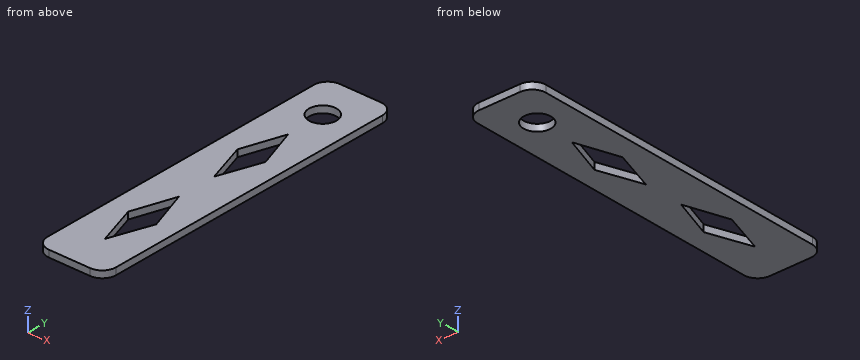
```python
from build123d import *

# Parameters (mm, degrees)
F0_R     = 12.7
F1_DEPTH = 6.35


with BuildPart() as f1:
    # F0 (on Top) → F1 (new body)
    with BuildSketch(Plane.XY):
        with BuildLine():
            ThreePointArc((0, 12.7), (3.719744, 3.719744), (12.7, 0))
            Line((12.7, 0), (50.8, 0))
            ThreePointArc((50.8, 0), (59.780256, 3.719744), (63.5, 12.7))
            Line((63.5, 12.7), (63.5, 292.1))
            ThreePointArc((63.5, 292.1), (59.780256, 301.080256), (50.8, 304.8))
            Line((50.8, 304.8), (12.7, 304.8))
            ThreePointArc((12.7, 304.8), (3.719744, 301.080256), (0, 292.1))
            Line((0, 292.1), (0, 12.7))
        make_face()
        Polygon((19.05, 75.692), (31.75, 114.540583), (45.188366, 75.692), (31.75, 36.843417), align=None, mode=Mode.SUBTRACT)
        Polygon((19.05, 190.246), (31.75, 229.094583), (45.188366, 190.246), (31.75, 151.397417), align=None, mode=Mode.SUBTRACT)
        with Locations((31.75, 265.397549)):
            Circle(F0_R, mode=Mode.SUBTRACT)
    extrude(amount=F1_DEPTH)


solid = f1.part
```
The listing builds one solid part. Answer for the finished solid, in the listing's coordinates (mm). Give positions to 0.01 mm unless a question says otherwise; leave off trailing zeros. Order: outer loops, then holes, each group sorted by start corner. A loop starts at its lowest first (then second) coordinate and runs counter-clockwise, first axis right, second up. Notation, with made-up numbers: (1, -38) -> (7, -38) arc R31 cw to (7, -13) -> close; hole circle Ø1 at (-32.5, -14). An arc over 180 degrees is marked (long way). Write each question's results on one line, items separated by ' | '.
Q1. The part is cut by section B-B, the plane y = 108.5. Give the vertices of the cut face in (x, z), and give its area (3 significant figures).
Checked values:
outline: (0, 0) -> (29.78, 0) -> (29.78, 6.35) -> (0, 6.35) -> close; (33.84, 0) -> (63.5, 0) -> (63.5, 6.35) -> (33.84, 6.35) -> close | area: 377 mm^2
Q2. Each of these flat-tipped pins is pushed along its axis until it touches: P1, Ø3, axis at x = 29.5, y = 53, coming from the +Z side; P2, Ø6, axis at x = 33.5, y = 100.5, coming from the -Z side; P3, Ø2, axis at x = 10, z = 1.5, coming from the -Y side. Where does it stop, or does it pass through?
Checked values:
P1: passes through | P2: stops at z = 0 | P3: stops at y = 0.11
Q3. The part is cut by section A-A, the plane x = 37. Give the vertices of the cut face in (y, z).
Checked values:
outline: (0, 0) -> (52.02, 0) -> (52.02, 6.35) -> (0, 6.35) -> close; (99.36, 0) -> (166.57, 0) -> (166.57, 6.35) -> (99.36, 6.35) -> close; (213.92, 0) -> (253.83, 0) -> (253.83, 6.35) -> (213.92, 6.35) -> close; (276.96, 0) -> (304.8, 0) -> (304.8, 6.35) -> (276.96, 6.35) -> close
Q4. The part is cut by section D-D, the plane y = 260. Give the vertices of the cut face in (x, z).
Checked values:
outline: (0, 0) -> (20.25, 0) -> (20.25, 6.35) -> (0, 6.35) -> close; (43.25, 0) -> (63.5, 0) -> (63.5, 6.35) -> (43.25, 6.35) -> close
Q5. Straight lines are drawn through the part: probe 1 along X at (y, z) = (196.5, 4) (1 decimal); probe 2 along X at (y, z) = (93, 5.75). For each, find the intervals that lie inside material, in ascending order. Write a range as from..to.
Checked values:
probe 1: x = 0..21.1, 43..63.5 | probe 2: x = 0..24.71, 39.2..63.5
Q6. The part is cut by section C-C, the plane z = 1.25. Give the vertices of the cut face in (x, y).
Checked values:
outline: (0, 12.7) arc R12.7 ccw to (12.7, 0) -> (50.8, 0) arc R12.7 ccw to (63.5, 12.7) -> (63.5, 292.1) arc R12.7 ccw to (50.8, 304.8) -> (12.7, 304.8) arc R12.7 ccw to (0, 292.1) -> close; hole (19.05, 75.69) -> (31.75, 36.84) -> (45.19, 75.69) -> (31.75, 114.54) -> close; hole (19.05, 190.25) -> (31.75, 151.4) -> (45.19, 190.25) -> (31.75, 229.09) -> close; hole circle Ø25.4 at (31.75, 265.4)
